The listing builds one solid part. Answer for the finished solid, in the listing's coordinates (mm). A direction names the side the tool comes from. Round coordinates to 2 decimals unless told otherwise and drop trailing zeros. Loops run counter-clockwise (first coordinate to the right, second up) from the corner with the lowest first, then second, coordinate; pieces in that order, holes last. Notation, with made-up numbers: (28.25, 68.25) -> (51.25, 68.25) arc R33 ccw to (51.25, 107.25) -> close; hole circle Ø11 at (36, 57). An arc over 180 degrees is marked (long way). One line per question, with ' | ' between items.
from build123d import *

# Parameters (mm, degrees)
SKETCH8_W              = 609.6
SKETCH8_H              = 174.625
BASE_FLANGE4_DEPTH     = 3.175
SKETCHED_START         = -304.8
SKETCHED_BEND4_DEPTH   = 609.6
SKETCHED_BEND4_2_DEPTH = 609.6
SKETCH24_W             = 609.6
SKETCH24_H             = 6.35
CUT_EXTRUDE1_DEPTH     = 328.356760899


# Read off the part's stored shape, not the designer's step: Sketched Bend4
# Sheet-metal steps are written as plain solids
with BuildPart() as part:
    # Sketch8 → Base-Flange4 (new body)
    with BuildSketch(Plane.XY):
        Rectangle(SKETCH8_W, SKETCH8_H)
    extrude(amount=-BASE_FLANGE4_DEPTH)

    # Sketched Bend4 outline → Sketched Bend4 (cut)
    with BuildSketch(Plane.YZ.offset(SKETCHED_START)):
        with BuildLine():
            ThreePointArc((-6.112156128, -3.175), (-8.604076071, -2.278520157), (-9.953774928, 0))
            Line((-9.953774928, 0), (-87.3125, 0))
            Line((-87.3125, 0), (-87.3125, -3.175))
            Line((-87.3125, -3.175), (-6.112156128, -3.175))
        make_face()
    extrude(amount=SKETCHED_BEND4_DEPTH, mode=Mode.SUBTRACT)

    # Sketched Bend4 2 outline → Sketched Bend4 2 (add)
    with BuildSketch(Plane.YZ.offset(SKETCHED_START)):
        with BuildLine():
            Line((-6.848756128, 78.286256128), (-10.023756128, 78.286256128))
            Line((-10.023756128, 78.286256128), (-10.023756128, 0.7366))
            ThreePointArc((-10.023756128, 0.7366), (-10.006221527, 0.366641581), (-9.953774928, 0))
            Line((-9.953774928, 0), (-6.112156128, 0))
            ThreePointArc((-6.112156128, 0), (-6.633010983, 0.215745145), (-6.848756128, 0.7366))
            Line((-6.848756128, 0.7366), (-6.848756128, 78.286256128))
        make_face()
    extrude(amount=SKETCHED_BEND4_2_DEPTH)

    # Sketch24 → Cut-Extrude1 (cut, through all)
    with BuildSketch(Plane(origin=(0, 0, -3.175), x_dir=(-1, 0, 0), z_dir=(0, 0, -1))):
        with Locations((0, 84.1375)):
            Rectangle(SKETCH24_W, SKETCH24_H)
    extrude(amount=-CUT_EXTRUDE1_DEPTH, mode=Mode.SUBTRACT)


solid = part.part
Q1. A cutting plane is placed at B-B on y = 52. Give the vertices of the cut face in (x, z) (3 decimals).
Numbers:
outline: (-304.8, -3.175) -> (304.8, -3.175) -> (304.8, 0) -> (-304.8, 0) -> close
Q2. A cutting plane is placed at C-C on z = 63. Give the vertices of the cut face in (x, y), plus the area to 3 significant figures.
Numbers:
outline: (-304.8, -10.02) -> (304.8, -10.02) -> (304.8, -6.85) -> (-304.8, -6.85) -> close | area: 1,940 mm^2
Q3. For faces 1 (the face through (-4, 38, 0)), 2 (the face through (-4, 38, -3.175)), determine the directions among +Z, -Z, +X, -X, +Y, -Y from which every point of the face is accessible in a straight line to the end or side of a thin tool.
Numbers:
face 1: +Z, +X, -X, +Y | face 2: -Z, +X, -X, +Y, -Y
Q4. A cutting plane is placed at A-A on x = -173. Give the vertices of the cut face in (y, z) (1 decimal).
Numbers:
outline: (-10, 0.7) arc R3.9 ccw to (-6.1, -3.2) -> (81, -3.2) -> (81, 0) -> (-6.1, 0) arc R0.7 cw to (-6.8, 0.7) -> (-6.8, 78.3) -> (-10, 78.3) -> close
Q5. Given pin 1 Ø8 at (x, y) = (-78, 31.5) entering from +Z, flat-ended and moving along its own axis, determine where the tip first touches the part or whether it passes through.
Numbers:
pin 1: z = 0
Q6. Find the intervals of material crossed by line 1 (Y direction, x = -199.5, z = 1); line 2 (Z direction, x = -7, y = 77.5) (3 decimals), in increasing order. Write a range as from..to.
Numbers:
line 1: -10.02..-6.85 | line 2: -3.175..0
